CAD build for the part. Positions are in the model's coordinates, mm. Face numbers are marked on the shaded views. A direction names the side the tool comes from. Coordinates: 2 decimals unless noted, no trailing zeros. Loops run counter-clockwise (first coordinate to the right, second up) from the corner with the lowest first, then second, coordinate; pieces in that order, holes last. Notation, with made-up numbers: (39, 32) -> (57, 32) arc R15 cw to (57, 39) -> close; hole circle Ø11 at (57, 30.5). An arc over 180 degrees is marked (long way). Write each question's results on one line, items separated by ' | '.
Autodesk Inventor part; units mm, degrees
ref_plane "YZ Plane" through (0, 0, 0) normal (1, 0, 0) x (0, 1, 0)
ref_plane "XZ Plane" through (0, 0, 0) normal (0, 1, 0) x (-1, 0, 0)
ref_plane "XY Plane" through (0, 0, 0) normal (0, 0, 1) x (1, 0, 0)
sketch "Sketch1" plane through (0, 0, 0) normal (1, 0, 0) x (0, 1, 0)
  line L0 (0, 0) -> (63.5, 0)
  line L1 (63.5, 0) -> (63.5, -63.5)
  line L2 (63.5, -63.5) -> (0, -63.5)
  line L3 (60.325, -3.175) -> (3.175, -3.175)
  line L4 (3.175, -60.325) -> (60.325, -60.325)
  line L5 (60.325, -60.325) -> (60.325, -3.175)
  line L6 (3.175, -3.175) -> (-12.9864, -3.175)
  line L7 (3.175, -60.325) -> (-8.5998, -60.325)
  line L8 (0, -63.5) -> (0, -60.325)
  line L9 (0, -3.175) -> (0, 0)
  dimension "d6" = 63.5
  dimension "d7" = 3.175
extrude "Extrusion1" add sketch "Sketch1" along normal blind 50.8
ref_plane "Work Plane1" through (0, 0, -31.75) normal (0, 0, -1) x (-1, 0, 0)
sketch "Sketch2" plane through (0, 0, 0) normal (0, 0, 1) x (1, 0, 0)
  line L0 (0, 0) -> (0, 63.5)
  line L1 (0, 63.5) -> (50.8, 63.5)
  line L2 (0, 0) -> (50.8, 0)
  point P0 (6.35, 15.875)
  dimension "d33" = 15.875
  dimension "d34" = 6.35
hole "Hole1" at (6.35, 15.875, 0) direction (0, 0, -1) diameter 6.35 end through all
sketch "Sketch4" plane through (0, 0, 0) normal (0, 0, 1) x (1, 0, 0)
  line L0 (50.8, 0) -> (50.8, 63.5)
  line L1 (50.8, 63.5) -> (34.925, 63.5)
  line L2 (34.925, 63.5) -> (34.925, 57.15)
  line L3 (50.8, 50.8) -> (50.8, 63.5)
  line L4 (50.8, 50.8) -> (34.925, 63.5)
  point P0 (0, 0)
  dimension "d58" = 15.875
  dimension "d60" = 12.7
extrude "Extrusion2" cut sketch "Sketch4" against normal through all
sketch "Sketch3" plane through (0, 0, 0) normal (0, 0, 1) x (1, 0, 0)
  circle A0 centre (6.35, 15.875) radius 3.175 construction
  line L0 (0, 0) -> (0, 63.5) construction
  line L1 (0, 0) -> (50.8, 0) construction
  line L2 (50.8, 50.8) -> (50.8, 0) construction
  line L3 (0, 63.5) -> (34.925, 63.5) construction
  line L4 (9.8817, -6.9679) -> (-8.7166, 33.4041) construction
  line L5 (-8.7166, 33.4041) -> (298.3815, 174.8763) construction
  line L6 (298.3815, 174.8763) -> (316.9799, 134.5042) construction
  line L7 (316.9799, 134.5042) -> (9.8817, -6.9679) construction
  line L8 (0, 60.325) -> (50.8, 60.325) construction
  line L9 (50.8, 50.8) -> (34.925, 63.5)
  point P0 (45.1543, 5.6457)
  point P1 (31.795, 55.5625)
  point P2 (288.925, 146.05)
  dimension "d36" = 6.35
  dimension "d38" = 5.6457
  dimension "d41" = 44.45
  dimension "d43" = 3.302
  dimension "d44" = 3.175
  dimension "d46" = 22.225
  dimension "d49" = 22.225
  dimension "d50" = 20.6502
  dimension "d52" = 130.175
  dimension "d53" = 4.7625
  dimension "d54" = 282.575
  dimension "d55" = 24.734
  dimension "d56" = 338.1178
  dimension "d57" = 5.6457
hole "Hole2" at (45.1543, 5.6457, 0) at (31.795, 55.5625, 0) direction (0, 0, -1) diameter 6.35 end through all
properties part number "CAR_024_KickerUChannel" material "Aluminum 6061"
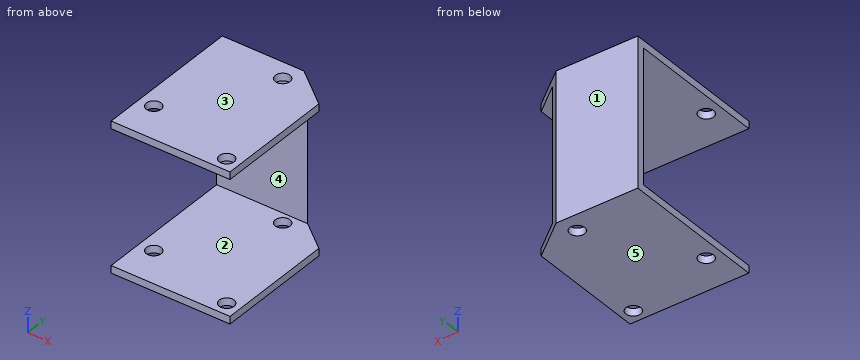
Q1. Cut at B-B on y = 25.5. Write the cut outline in (x, z) (3 decimals), and give its area (3 significant figures).
Results are:
outline: (0, -63.5) -> (50.8, -63.5) -> (50.8, -60.325) -> (0, -60.325) -> close; (0, -3.175) -> (50.8, -3.175) -> (50.8, 0) -> (0, 0) -> close | area: 323 mm^2
Q2. Cut at D-D on z = -53.5. Write the cut outline in (x, y) (3 decimals).
Results are:
outline: (0, 60.325) -> (38.894, 60.325) -> (34.925, 63.5) -> (0, 63.5) -> close
Q3. Cut at C-C on x = 17. Write the cut outline in (y, z) (3 decimals), and give its area (3 significant figures).
Results are:
outline: (0, -63.5) -> (63.5, -63.5) -> (63.5, 0) -> (0, 0) -> (0, -3.175) -> (60.325, -3.175) -> (60.325, -60.325) -> (0, -60.325) -> close | area: 585 mm^2
Q4. Drop flat-ended pins along their axis: pin 1 (5.5 mm diameter, centred on x = 45.15, y = 5.65, fed in from -Z); pin 2 (8.5 mm diameter, centred on x = 31.8, y = 55.56, fed in from -Z); pin 3 (11.5 mm diameter, centred on x = 27, z = -43.5, fed in from -Y) (3 decimals). Give the stop position or say it passes through.
Results are:
pin 1: through | pin 2: z = -63.5 | pin 3: y = 60.325
Q5. Cut at A-A on x = 6.35. Write the cut outline in (y, z) (3 decimals).
Results are:
outline: (0, -63.5) -> (12.7, -63.5) -> (12.7, -60.325) -> (0, -60.325) -> close; (0, -3.175) -> (12.7, -3.175) -> (12.7, 0) -> (0, 0) -> close; (19.05, -63.5) -> (63.5, -63.5) -> (63.5, 0) -> (19.05, 0) -> (19.05, -3.175) -> (60.325, -3.175) -> (60.325, -60.325) -> (19.05, -60.325) -> close
Q6. Wall check: L1, parallel to Z at x = 36, y = 42 (3 decimals); L2, parallel to Y at x = 6.5, z = -33 (3 decimals); L3, parallel to Y at x = 36.5, z = -28 (3 decimals). Give the ranges that are in metal, low to high. Write a range as from..to.
Results are:
L1: -63.5..-60.325, -3.175..0 | L2: 60.325..63.5 | L3: 60.325..62.24
Q7. Pull direction Z, two halves, no side cores. Call the marked faces 1, 2 and 3: +Z half, -Z half, draft (parallel to the pull), parting line (faces both ways), or undercut.
Results are:
face 1: draft | face 2: undercut | face 3: +Z half
Q8. Which spindle directions (+Z, -Z, +X, -X, +Y, -Y) get a long thin tool onto all of the face, cutting with end or side? Do the marked faces 4 and 5. Say none if no direction does.
Results are:
face 4: +X, -X, -Y | face 5: -Z, +X, -X, +Y, -Y
